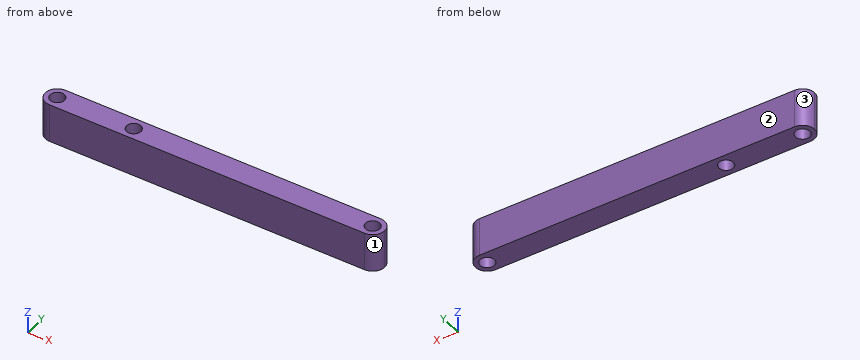
```python
from build123d import *

# Parameters (mm, degrees)
F0_W     = 225.425
F0_H     = 15.875
F1_DEPTH = 25.4
F3_D     = 9.525
F4_R     = 7.93749


# Not quite as in the source:
# - a fillet or chamfer is up to 0.001 mm smaller than in the source, because OpenCascade refuses the exact size


with BuildPart() as f1:
    # F0 (on Top) → F1 (new body)
    with BuildSketch(Plane.XY):
        Rectangle(F0_W, F0_H)
    extrude(amount=F1_DEPTH)

    # F3 (through all)
    with Locations(Plane.XY.offset(25.4)):
        with Locations((104.775, 0), (-104.775, 0), (-53.975, 0)):
            Hole(F3_D / 2)

    # F4 (radius 7.9375 in the source; OpenCascade refuses exactly that, so slightly less here)
    f4_edges = [f1.edges().sort_by_distance(p)[0] for p in [
        (-112.7125, -7.9375, 12.7),
        (112.7125, -7.9375, 12.7),
        (112.7125, 7.9375, 12.7),
        (-112.7125, 7.9375, 12.7),
    ]]
    fillet(f4_edges, radius=F4_R)


solid = f1.part
```
Source: CAD feature listing. Evaluate the final solid. Frame: model axes, mm. Face numbers are marked on the shaded views. Round coordinates to 2 decimals unless told otherwise and drop trailing zeros. Use CSV: the item, a comma, the result in double quotes. Start each with the question number.
Q1. Cut plane A-A on z = 17.5. Count the separate pieces of the cut face and the enclosed holes in it, plus the area to 3 significant figures.
Q2. Pull-direction query (X, two-part tool) for the marked faces 1, 2 and 3; classes: +X half, -X half, draft (parallel to the pull), parting line (faces both ways), or undercut.
Q3. Line query: line 1 (X direction, y = 2.5, z = 7.75); line 2 (X direction, y = -4.25, z = 2.25); line 3 (Y direction, x = -50, z = 16). Output: solid intervals per line, ascending. Write a range as from..to.
Q4. First-contact query: P1, Ø6, axis at y = 5.5, z = 3, coming from the -X side; P2, Ø8.5, axis at x = -104.775, y = 0, coming from the +Z side; P3, Ø1.5, axis at y = 4, z = 23, coming from the -X side. Flat tips, straight axial feed; report the tip coordinate or a pass-through.
Results found:
1,separate pieces,"1"
1,enclosed holes,"3"
1,area,"3,310 mm^2"
2,face 1,"+X half"
2,face 2,"draft"
2,face 3,"-X half"
3,line 1,"-112.31..-108.83, -100.72..-58.03, -49.92..100.72, 108.83..112.31"
3,line 2,"-111.48..-106.92, -102.63..-56.12, -51.83..102.63, 106.92..111.48"
3,line 3,"-7.94..-2.62, 2.62..7.94"
4,P1,"x = -112.31"
4,P2,"through"
4,P3,"x = -112.02"
